Autodesk Inventor part; units mm, degrees
ref_plane "YZ Plane" through (0, 0, 0) normal (1, 0, 0) x (0, 1, 0)
ref_plane "XZ Plane" through (0, 0, 0) normal (0, 1, 0) x (-1, 0, 0)
ref_plane "XY Plane" through (0, 0, 0) normal (0, 0, 1) x (1, 0, 0)
sketch "Sketch1" plane through (0, 0, 0) normal (0, 1, 0) x (-1, 0, 0)
  line L0 (0, 0) -> (140, 0)
  line L1 (140, 0) -> (140, -170)
  line L2 (140, -170) -> (0, -170)
  line L3 (0, -170) -> (0, 0)
  line L4 (140, 0) -> (137.5, 0)
  line L5 (140, -2.5) -> (140, 0)
  line L6 (140, -170) -> (135, -170)
  line L7 (135, -170) -> (135, -165)
  line L8 (135, -165) -> (140, -165)
  line L9 (140, -165) -> (140, -170)
  circle A0 centre (135, -165) radius 2
  line L10 (0, 0) -> (5, 0)
  line L11 (5, 0) -> (5, -5)
  line L12 (5, -5) -> (0, -5)
  line L13 (0, -5) -> (0, 0)
  circle A1 centre (5, -5) radius 2
  circle A2 centre (5, -165) radius 2
  circle A3 centre (135, -5) radius 2
  dimension "d0" = 140
  dimension "d1" = 170
  dimension "d25" = 5
  dimension "d26" = 5
  dimension "d27" = 4
  dimension "d28" = 5
  dimension "d29" = 5
  dimension "d30" = 4
  dimension "d31" = 4
  dimension "d32" = 4
extrude "Extrusion5" add sketch "Sketch1" along normal blind 3 contours L0 L11 A1 L12 L3 | L0 L1 L8 A0 L7 L2 L3 L12 A1 L11 | L7 A0 L8 L1 L2
sketch "Sketch5" plane through (0, 3, 0) normal (0, 1, 0) x (1, 0, 0)
  line L0 (0, 170) -> (-140, 170)
  circle A0 centre (-70, 100) radius 41
  point P0 (0, 0)
  dimension "d36" = 82
extrude "Extrusion6" cut sketch "Sketch5" against normal blind 10
sketch "Sketch6" plane through (0, 3, 0) normal (0, 1, 0) x (1, 0, 0)
  circle A0 centre (-70, 100) radius 41
  circle A1 centre (-70, 100) radius 41
  circle A2 centre (-70, 100) radius 42
  point P0 (0, 0)
  dimension "d39" = 84
extrude "Extrusion7" cut sketch "Sketch6" against normal blind 2
properties part number "back"
The listing builds one solid part. Answer for the finished solid, in the listing's coordinates (mm). A direction names the side the tool comes from. Coordinates: 2 decimals unless noted, no trailing zeros. Write each loop counter-clockwise with the first axis right and the second up, starting at its lowest first coordinate (ties: lowest second). Pieces come first, ordered by that corner, then holes. Notation, with made-up numbers: (14.5, -30.5) - (56.5, -30.5) arc R18 ccw to (56.5, -4.5) - close; hole circle Ø6 at (42.5, 75). An arc over 180 degrees is marked (long way). Return JSON: item names as keys, results as strings.
1. For a pull along Z with two mould halves and no side action, classify faces 1 (the face through (-29.8, 1, -90.9)), 2 (the face through (-69, 3, -46)) as +Z half, -Z half, draft (parallel to the pull), parting line (faces both ways), or undercut.
Final values:
{"face 1": "undercut", "face 2": "draft"}
2. This flat-tipped pin is pushed along its axis until it touches: pin 1 Ø2.5 at (x, z) = (-135, -165) entering from +Y. Where does it stop, or does it pass through?
Final values:
{"pin 1": "through"}
3. Which of the six approach directions +Z, -Z, +X, -X, +Y, -Y give full straight-line access (tool end or side, diameter ignored) to faces 3 (the face through (-47.4, 2, -135.4)), 4 (the face through (-5.923, 1.479, -163.226))?
Final values:
{"face 3": "+Y", "face 4": "+Y, -Y"}
4. The part is cut by section D-D on x = -70. Determine the outline of the cut face in (y, z), then the cut area to 3 significant figures.
Final values:
{"outline": "(0, -170) - (3, -170) - (3, -142) - (1, -142) - (1, -141) - (0, -141) - close; (0, -59) - (1, -59) - (1, -58) - (3, -58) - (3, 0) - (0, 0) - close", "area": "260 mm^2"}
5. The part is cut by section C-C on z = -165. Determine the outline of the cut face in (x, y).
Final values:
{"outline": "(-140, 0) - (-137, 0) - (-137, 3) - (-140, 3) - close; (-133, 0) - (-7, 0) - (-7, 3) - (-133, 3) - close; (-3, 0) - (0, 0) - (0, 3) - (-3, 3) - close"}
6. Consider line 1 along Z through (x, y) = (-5, 2); line 2 along X through (y, z) = (1.6, -165); line 3 along Z through (x, y) = (-70, 0.7). Determine where each line is inside the solid, lowest interval first.
Final values:
{"line 1": "-170 to -167, -163 to -7, -3 to 0", "line 2": "-140 to -137, -133 to -7, -3 to 0", "line 3": "-170 to -141, -59 to 0"}
7. The part is cut by section B-B on y = 0.45. Determine the outline of the cut face in (x, z), then the cut area to 3 significant figures.
Final values:
{"outline": "(-140, -170) - (0, -170) - (0, 0) - (-140, 0) - close; hole circle Ø4 at (-135, -165); hole circle Ø4 at (-135, -5); hole circle Ø82 at (-70, -100); hole circle Ø4 at (-5, -165); hole circle Ø4 at (-5, -5)", "area": "18,500 mm^2"}
8. The part is cut by section A-A on x = -5. Determine the outline of the cut face in (y, z).
Final values:
{"outline": "(0, -170) - (3, -170) - (3, -167) - (0, -167) - close; (0, -163) - (3, -163) - (3, -7) - (0, -7) - close; (0, -3) - (3, -3) - (3, 0) - (0, 0) - close"}
